from build123d import *

# Parameters (mm, degrees)
SKETCH2_R           = 4.25
SKETCH2_R_2         = 2
BOSS_EXTRUDE1_DEPTH = 5
SKETCH_1_R          = 1.75
CUT_EXTRUDE_1_DEPTH = 10


with BuildPart() as part:
    # Sketch2 → Boss-Extrude1 (new body)
    with BuildSketch(Plane.XY):
        with BuildLine():
            Line((-17.328874887, 74.839530577), (33.78000003, 66.278338859))
            ThreePointArc((33.78000003, 66.278338859), (42.753857637, 57.963816533), (35.14697315, 48.382756557))
            Line((35.14697315, 48.382756557), (-17.561996681, 40.283034413))
            ThreePointArc((-17.561996681, 40.283034413), (-37.719601772, 57.698054173), (-17.328874887, 74.839530577))
        make_face()
        with Locations((-20.21999997, 57.58)):
            Circle(SKETCH2_R, mode=Mode.SUBTRACT)
        with Locations((33.78000003, 57.278338859)):
            Circle(SKETCH2_R_2, mode=Mode.SUBTRACT)
    extrude(amount=-BOSS_EXTRUDE1_DEPTH)

    # 草图1 → 切除-拉伸1 (cut)
    with BuildSketch(Plane.XY):
        with Locations((-13.21999997, 57.58)):
            Circle(SKETCH_1_R)
        with Locations((-27.21999997, 57.58)):
            Circle(SKETCH_1_R)
        with Locations((-20.21999997, 64.58)):
            Circle(SKETCH_1_R)
        with Locations((-20.21999997, 50.58)):
            Circle(SKETCH_1_R)
    extrude(amount=-CUT_EXTRUDE_1_DEPTH, mode=Mode.SUBTRACT)


solid = part.part
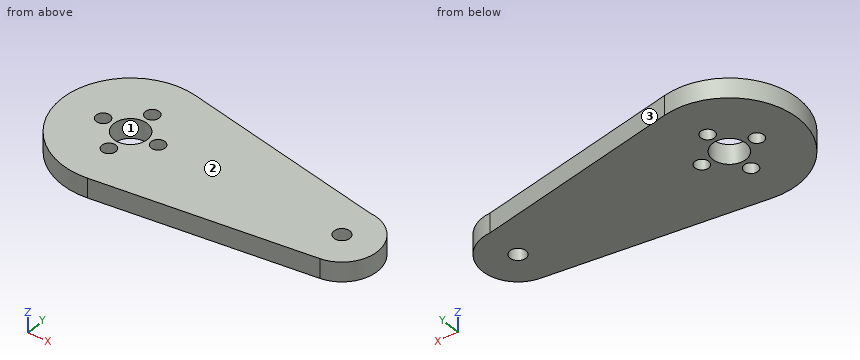
Design review of the part built by this model. Coordinates are the model's own, in mm. Face numbers are marked on the shaded views. Round coordinates to 2 decimals unless told otherwise and drop trailing zeros. Write each loop counter-clockwise with the first axis right and the second up, starting at its lowest first coordinate (ties: lowest second). Pieces come first, ordered by that corner, then holes. Notation, with made-up numbers: (87.25, 88) -> (146.25, 88) arc R25 cw to (146.25, 108) -> close; hole circle Ø4 at (37, -19). An arc over 180 degrees is marked (long way). One line per item, written item: value. Start each with the question number.
Q1. The part is to be moulded in two halves that separate along X. For the marked faces 1, 2 and 3, say which applies: pulls with the +X half, pulls with the -X half, needs draft (parallel to the pull), parting line crosses it, or undercut.
Q2. Insertion check: P1, Ø2, axis at x = 0.5, z = -3.5, coming from the -Y side; P2, Ø1.5, axis at x = -24, z = -2, coming from the -Y side. Each pin has a flat end and moves straight along its axis. Give the tip position at first contact, or say it passes through.
Q3. To check wall thickness, follow probe 1 along X at (y, z) = (59, -1.95); probe 2 along X at (y, z) = (56, -3.7); probe 3 along Y at (x, z) = (-13.22, -2.7). State the ranges of each line that lie inside material, in increasing order.
Q4. Add section D-D (x = 23). Give the boundary of the cut face in (y, z).
Q5. Add section B-B (y = 50.58). Give the boundary of the cut face in (x, z), then the cut area to 3 significant figures.
Q6. Add section C-C (z = -2.6). Give the boundary of the cut face in (x, y), then the cut area to 3 significant figures.
Q7. Add section A-A (x = -13.22). Give the boundary of the cut face in (y, z).
Response:
1. face 1: undercut
1. face 2: needs draft
1. face 3: pulls with the +X half
2. P1: stops at y = 42.9
2. P2: stops at y = 40.34
3. probe 1: x = -37.66 to -28.24, -26.2 to -24.23, -16.21 to -14.24, -12.2 to 32.76, 34.8 to 42.61
3. probe 2: x = -37.65 to -27.97, -26.47 to -24.17, -16.27 to -13.97, -12.47 to 32.24, 35.32 to 42.69
3. probe 3: y = 40.95 to 55.83, 59.33 to 74.15
4. outline: (46.52, -5) -> (68.08, -5) -> (68.08, 0) -> (46.52, 0) -> close
5. outline: (-36.26, -5) -> (-21.97, -5) -> (-21.97, 0) -> (-36.26, 0) -> close; (-18.47, -5) -> (39.79, -5) -> (39.79, 0) -> (-18.47, 0) -> close
5. area: 363 mm^2
6. outline: (-17.56, 40.28) -> (35.15, 48.38) arc R9 ccw to (33.78, 66.28) -> (-17.33, 74.84) arc R17.5 ccw (long way) to start; hole circle Ø3.5 at (-27.22, 57.58); hole circle Ø8.5 at (-20.22, 57.58); hole circle Ø3.5 at (-20.22, 50.58); hole circle Ø3.5 at (-20.22, 64.58); hole circle Ø3.5 at (-13.22, 57.58); hole circle Ø4 at (33.78, 57.28)
6. area: 1,950 mm^2
7. outline: (40.95, -5) -> (55.83, -5) -> (55.83, 0) -> (40.95, 0) -> close; (59.33, -5) -> (74.15, -5) -> (74.15, 0) -> (59.33, 0) -> close
